Check sheet for the modelled part. Datum: model origin and axes. Units: mm. Round coordinates to 2 decimals unless told otherwise and drop trailing zeros. Loops run counter-clockwise (first coordinate to the right, second up) from the corner with the lowest first, then second, coordinate; pieces in that order, holes last. Notation, with made-up numbers: M -20,-35 L -14,-35 A23 ccw -14,-10 Z; hole C 86,24.25 d5. An arc over 180 degrees is marked long. Write item = value, one per line. Start each with the question number.
(1) Cross-section at C-C on x = 7. Record the boundary of the cut face in (y, z).
(2) Cross-section at D-D on z = 37. Record the boundary of the cut face in (x, y).
(3) Mould release check, pull along X, two halves, no side actions. Record for faces 1 (the face through (43.14, 4.56, 0.9)), 2 (the face through (7.07, 4.56, 35.35)), 3 (the face through (22, 5, 44)): pulls with the +X half, pulls with the -X half, needs draft (parallel to the pull), parting line crosses it, or undercut.
(4) Scan lines: L1, parallel to X at y = 2.5, z = 7; L2, parallel to Z at x = 38, y = 5; L3, parallel to Z at x = 36.5, y = 5.25. Record each from-to range of solid material in increasing order. Write a range as from..to.
(5) Cross-section at A-A on x = 22. Record the boundary of the cut face in (y, z), plus the area to 3 significant figures.
(6) Cross-section at B-B on z = 22. Record the boundary of the cut face in (x, y).
from build123d import *

# Parameters (mm, degrees)
SKETCH_1_W          = 44
SKETCH_1_H          = 9
RAISED_FLANGE_DEPTH = 44
FILLET_2_R          = 3
SKETCH_2_R          = 8.3
FLANGE_HOLE_DEPTH   = 63.872887638
SKETCH_3_R          = 1.65
CUT_EXTRUDE_2_DEPTH = 63.872887638
SKETCH_4_R          = 1.65
CUT_EXTRUDE_3_DEPTH = 63.872887638
SKETCH_5_R          = 1.65
CUT_EXTRUDE_4_DEPTH = 63.872887638
SKETCH_6_R          = 1.65
CUT_EXTRUDE_5_DEPTH = 63.872887638


with BuildPart() as part:
    # 草图1 → Raised_flange (new body)
    with BuildSketch(Plane.XY):
        with Locations((22, 4.5)):
            Rectangle(SKETCH_1_W, SKETCH_1_H)
    extrude(amount=RAISED_FLANGE_DEPTH)

    # Fillet 2
    fillet_2_edges = [part.edges().sort_by_distance(p)[0] for p in [
        (44, 4.5, 44),
        (0, 4.5, 44),
        (44, 4.5, 0),
        (0, 4.5, 0),
    ]]
    fillet(fillet_2_edges, radius=FILLET_2_R)

    # 草图2 → Flange_hole (cut, through all)
    with BuildSketch(Plane(origin=(0, 9, 0), x_dir=(1, 0, 0), z_dir=(0, 1, 0))):
        with Locations(Location((22, -22, 0), (0, 0, 270))):
            Circle(SKETCH_2_R)
    extrude(amount=-FLANGE_HOLE_DEPTH, mode=Mode.SUBTRACT)

    # 草图3 → 切除-拉伸2 (cut, through all)
    with BuildSketch(Plane(origin=(0, 9, 0), x_dir=(1, 0, 0), z_dir=(0, 1, 0))):
        with Locations(Location((7, -7, 0), (0, 0, 270))):
            Circle(SKETCH_3_R)
    extrude(amount=-CUT_EXTRUDE_2_DEPTH, mode=Mode.SUBTRACT)

    # 草图4 → 切除-拉伸3 (cut, through all)
    with BuildSketch(Plane(origin=(0, 9, 0), x_dir=(1, 0, 0), z_dir=(0, 1, 0))):
        with Locations(Location((7, -37, 0), (0, 0, 270))):
            Circle(SKETCH_4_R)
    extrude(amount=-CUT_EXTRUDE_3_DEPTH, mode=Mode.SUBTRACT)

    # 草图5 → 切除-拉伸4 (cut, through all)
    with BuildSketch(Plane(origin=(0, 9, 0), x_dir=(1, 0, 0), z_dir=(0, 1, 0))):
        with Locations(Location((37, -7, 0), (0, 0, 270))):
            Circle(SKETCH_5_R)
    extrude(amount=-CUT_EXTRUDE_4_DEPTH, mode=Mode.SUBTRACT)

    # 草图6 → 切除-拉伸5 (cut, through all)
    with BuildSketch(Plane(origin=(0, 9, 0), x_dir=(1, 0, 0), z_dir=(0, 1, 0))):
        with Locations(Location((37, -37, 0), (0, 0, 270))):
            Circle(SKETCH_6_R)
    extrude(amount=-CUT_EXTRUDE_5_DEPTH, mode=Mode.SUBTRACT)


solid = part.part
Result:
q1.outline = M 0,0 L 9,0 L 9,5.35 L 0,5.35 Z; M 0,8.65 L 9,8.65 L 9,35.35 L 0,35.35 Z; M 0,38.65 L 9,38.65 L 9,44 L 0,44 Z
q2.outline = M 0,0 L 5.35,0 L 5.35,9 L 0,9 Z; M 8.65,0 L 35.35,0 L 35.35,9 L 8.65,9 Z; M 38.65,0 L 44,0 L 44,9 L 38.65,9 Z
q3.face_1 = pulls with the +X half
q3.face_2 = undercut
q3.face_3 = needs draft
q4.L1 = 0..5.35, 8.65..35.35, 38.65..44
q4.L2 = 0..5.69, 8.31..35.69, 38.31..44
q4.L3 = 0..5.43, 8.57..35.43, 38.57..44
q5.outline = M 0,0 L 9,0 L 9,13.7 L 0,13.7 Z; M 0,30.3 L 9,30.3 L 9,44 L 0,44 Z
q5.area = 247 mm^2
q6.outline = M 0,0 L 13.7,0 L 13.7,9 L 0,9 Z; M 30.3,0 L 44,0 L 44,9 L 30.3,9 Z
